The listing builds one solid part. Answer for the finished solid, in the listing's coordinates (mm). Give positions to 0.01 mm unless a question says otherwise; leave off trailing zeros. Loops run counter-clockwise (first coordinate to the right, second up) from the corner with the lowest first, then second, coordinate; pieces in that order, holes last. Notation, with made-up numbers: M -39.5,-13.75 L -19.5,-13.75 A20 cw -19.5,6.25 Z; hole C 81.5,-4 d10. An arc over 180 degrees is marked long. Return JSON: item names as keys, results as strings.
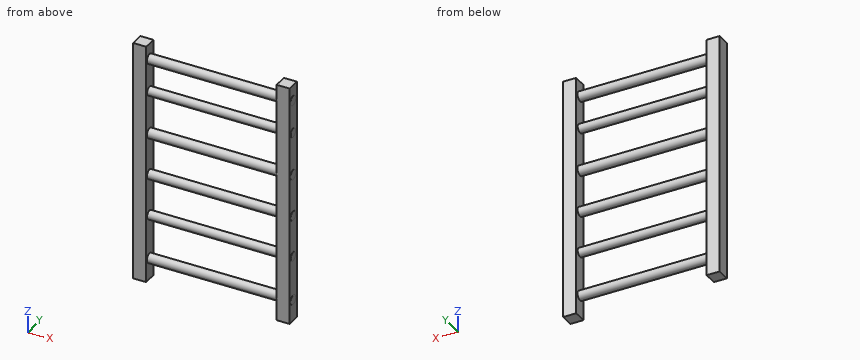
from build123d import *

# Parameters (mm, degrees)
F0_W     = 38.1
F0_H     = 711.2
F1_DEPTH = 38.1
F2_R     = 14.0648438742
F2_R_2   = 12.8526687622
F2_R_3   = 14.3519624693
F2_R_4   = 13.5478861372
F2_R_5   = 12.852653861
F2_R_6   = 13.899417222
F3_DEPTH = 457.2


with BuildPart() as f1:
    # F0 (on Front) → F1 (new body)
    with BuildSketch(Plane.XZ):
        with Locations((-112.7485206842, 291.7568912864)):
            Rectangle(F0_W, F0_H)
    extrude(amount=F1_DEPTH)



with BuildPart() as f1b:
    # F0 (on Front) → F1, piece 2 (new body)
    with BuildSketch(Plane.XZ):
        with Locations((305.7854154587, 291.7568912864)):
            Rectangle(F0_W, F0_H)
    extrude(amount=F1_DEPTH)


with BuildPart() as f1_1:
    add(f1.part)

    add(f1b.part)  # F3 merges F1b
    # F2 (on face) → F3 (join)
    with BuildSketch(Plane(origin=(-131.7985206842, 0, 0), x_dir=(0, -1, 0), z_dir=(-1, 0, 0))):
        with Locations((20.7070652395, 601.8965244293)):
            Circle(F2_R)
        with Locations((20.7070652395, 504.7876238823)):
            Circle(F2_R_2)
        with Locations((20.7070652395, 377.6891231537)):
            Circle(F2_R_3)
        with Locations((20.7070652395, 253.4467875957)):
            Circle(F2_R_4)
        with Locations((20.7070652395, 130.6325346231)):
            Circle(F2_R_5)
        with Locations((20.7070652395, 0)):
            Circle(F2_R_6)
    extrude(amount=-F3_DEPTH)


solid = f1_1.part
(1) The part is cut by section B-B (z = 0). Determine the outline of the cut face in (x, y).
Values follow:
{"outline": "M -131.8,-38.1 L -93.7,-38.1 L -93.7,-34.61 L 286.74,-34.61 L 286.74,-38.1 L 324.84,-38.1 L 324.84,-34.61 L 325.4,-34.61 L 325.4,-6.81 L 324.84,-6.81 L 324.84,0 L 286.74,0 L 286.74,-6.81 L -93.7,-6.81 L -93.7,0 L -131.8,0 Z"}
(2) Straight lines are drawn through the part: line 1 along X through (y, z) = (-35.5, 238); line 2 along Z through (x, y) = (160.5, -11.5); line 3 along Z through (x, y) = (156.5, -19.5). For each, find the intervals that lie inside material, in ascending order.
Values follow:
{"line 1": "-131.8 to -93.7, 286.74 to 324.84", "line 2": "-10.41 to 10.41, 121.66 to 139.6, 243.51 to 263.39, 366.68 to 388.7, 495.82 to 513.76, 591.26 to 612.53", "line 3": "-13.85 to 13.85, 117.84 to 143.43, 239.95 to 266.94, 363.39 to 391.99, 491.99 to 517.58, 587.88 to 615.91"}
(3) The part is cut by section A-A (z = 152). Determine the outline of the cut face in (x, y).
Values follow:
{"outline": "M -131.8,-38.1 L -93.7,-38.1 L -93.7,0 L -131.8,0 Z; M 286.74,-38.1 L 324.84,-38.1 L 324.84,0 L 286.74,0 Z"}
(4) The part is cut by section C-C (x = 228). Determine the outline of the cut face in (y, z), and give its area (3 significant figures).
Values follow:
{"outline": "C -20.71,377.69 d28.7; C -20.71,601.9 d28.13; C -20.71,0 d27.8; C -20.71,253.45 d27.1; C -20.71,130.63 d25.71; C -20.71,504.79 d25.71", "area": "3,490 mm²"}
(5) Given pin 1 (8 mm diameter, centred on x = -3, y = -20.5, fed in from -Z); pin 2 (19 mm diameter, centred on y = -23, z = 225.5, fed in from +X); pin 3 (1 mm diameter, centred on x = 134, y = -22, fed in from +Z), each flat-ended and moving along its own axis, determine where each tip first touches the part or whether it passes through.
Values follow:
{"pin 1": "z = -13.9", "pin 2": "x = 324.84", "pin 3": "z = 615.94"}
(6) The part is cut by section D-D (y = -18.5). Give the number of separate pieces and of enclosed holes in the cut face, and give its area (3 significant figures).
Values follow:
{"separate pieces": "1", "enclosed holes": "5", "area": "116,000 mm²"}
